Read the model definition and answer for the solid it produces. Units are mm, in the model's axes. A direction names the side the tool comes from. Coordinates: 2 decimals unless noted, no trailing zeros. Write each loop counter-clockwise with the first axis right and the second up, starting at its lowest first coordinate (ties: lowest second). Pieces come first, ordered by that corner, then holes.
(1) Given pin 1 (3 mm diameter, centred on x = 50, y = -15.5, fed in from +Z); pin 2 (11 mm diameter, centred on x = -20, y = -24.5, fed in from -Z); pin 3 (5 mm diameter, centred on y = -9.5, z = -27, fed in from +X), each flat-ended and moving along its own axis, determine where each tip first touches the part or whether it passes through.
(2) Which of the six approach directions +Z, -Z, +X, -X, +Y, -Y give full straight-line access (tool end or side, diameter ignored) to faces 4 (the cylindrical face through (-11.69, -1.53, -36.46)), 5 (the cylindrical face through (2.05, -1.53, 36.46))?
(3) Determine the mould class of faces 1 (the flat face through (21, -41.656, -6)), 2 (the cylindrical face through (-35.772, -1.528, -0.46)), 3 (the cylindrical face through (37.28, -21.12, -5.49)) for opening direction X: pulls with the +X half, pulls with the -X half, needs draft (parallel to the pull), parting line crosses it, or undercut.
(4) Straight lines are drawn through the part: line 1 along Z through (x, y) = (0.5, -34); line 2 along Z through (x, y) = (37, -18.5); line 3 along Z through (x, y) = (43, -28). For each, find the intervals that lie inside material, in ascending order.
(5) The part is cut by section A-A, the plane y = -31. Determine the outline of the cut face in (x, z), and give its area (3 significant figures).
```python
from build123d import *

# Parameters (mm, degrees)
F1_DEPTH = 41.656
F2_R     = 5.08
F3_R     = 7.781116
F4_DEPTH = 55.626


with BuildPart() as f1:
    # F0 (on Front) → F1 (new body)
    with BuildSketch(Plane.XZ):
        with BuildLine():
            Line((37.220769, -37.904616), (37.220769, 37.904616))
            ThreePointArc((37.220769, 37.904616), (-3.764667, 10.445012), (6.040904, -37.904616))
            Line((6.040904, -37.904616), (37.220769, -37.904616))
        make_face()
        with BuildLine():
            ThreePointArc((81.537427, -6.412042), (68.557378, 24.924568), (37.220769, 37.904616))
            Line((37.220769, 37.904616), (37.220769, -37.904616))
            Line((37.220769, -37.904616), (6.040904, -37.904616))
            ThreePointArc((6.040904, -37.904616), (54.282111, -47.312858), (81.537427, -6.412042))
        make_face()
        with BuildLine():
            Line((37.220769, 37.904616), (-37.220769, 37.904616))
            Line((-37.220769, 37.904616), (-37.220769, -37.904616))
            Line((-37.220769, -37.904616), (6.040904, -37.904616))
            ThreePointArc((6.040904, -37.904616), (-3.764667, 10.445012), (37.220769, 37.904616))
        make_face()
    extrude(amount=F1_DEPTH)

    # F2
    f2_edges = [f1.edges().sort_by_distance(p)[0] for p in [
        (0, -41.656, 37.904616),
        (37.220769, -20.828, 37.904616),
        (78.206204, 0, -23.269096),
        (-15.589932, 0, -37.904616),
        (-37.220769, 0, 0),
        (-37.220769, -20.828, 37.904616),
        (-37.220769, -41.656, 0),
        (-37.220769, -20.828, -37.904616),
    ]]
    fillet(f2_edges, radius=F2_R)

    # F3 (on face) → F4 (cut)
    with BuildSketch(Plane.XZ.offset(41.656)):
        with Locations((43.015637, -10.746155)):
            Circle(F3_R)
    extrude(amount=-F4_DEPTH, mode=Mode.SUBTRACT)


solid = f1.part
```
Computed:
1. pin 1: stops at z = 36.45
1. pin 2: stops at z = -37.9
1. pin 3: stops at x = 77.68
2. face 4: -Z, -X, +Y
2. face 5: +Z, +X, -X, +Y
3. face 1: needs draft
3. face 2: pulls with the -X half
3. face 3: undercut
4. line 1: z = -37.9 to 37.9
4. line 2: z = -50.73 to -15.68, -5.81 to 37.9
4. line 3: z = -50.35 to -18.53, -2.97 to 37.53
5. outline: (-37.22, -32.82) arc R5.08 ccw to (-32.14, -37.9) - (6.04, -37.9) arc R44.32 ccw (long way) to (37.22, 37.9) - (-32.14, 37.9) arc R5.08 ccw to (-37.22, 32.82) - close; hole circle Ø15.56 at (43.02, -10.75)
5. area: 8,800 mm2
